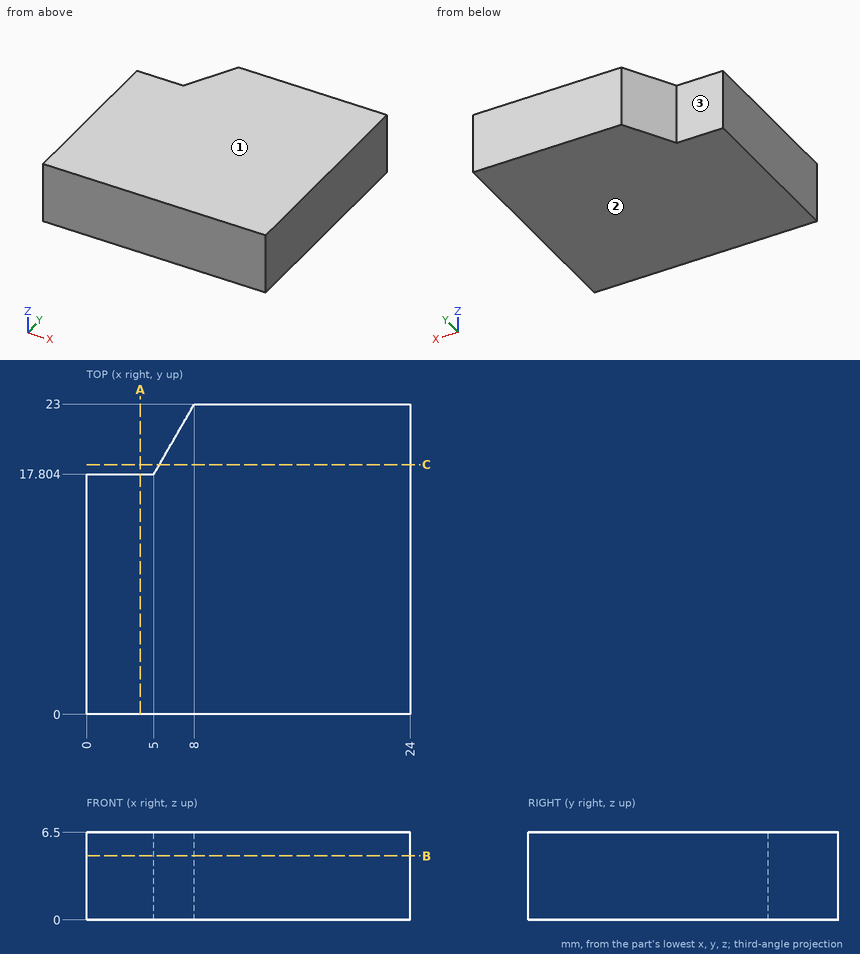
Verification items for this drawing (mm, ordinates from the low corner). Give positions to 0.01 mm unless a question says otherwise; leave off trailing zeros. Loops run counter-clockwise (first coordinate to the right, second up) from the corner with the lowest first, then second, coordinate; pieces in that order, holes last.
(1) Release check for a two-part mould opening along Z. For the marked faces 1, 2 and 3 record: released by +Z, released by -Z, zero draft, split by the parting line, or undercut.
From the geometry:
face 1: released by +Z
face 2: released by -Z
face 3: zero draft
(2) Section check C-C on y = 18.5. Record the cut outline in (x, z), then the cut area to 3 significant figures.
From the geometry:
outline: (5.4, 0) - (24, 0) - (24, 6.5) - (5.4, 6.5) - close
area: 121 mm2
(3) Section check A-A on x = 4. Record the cut outline in (y, z).
From the geometry:
outline: (0, 0) - (17.8, 0) - (17.8, 6.5) - (0, 6.5) - close
(4) Section check B-B on z = 4.75. Record the cut outline in (x, y).
From the geometry:
outline: (0, 0) - (24, 0) - (24, 23) - (8, 23) - (5, 17.8) - (0, 17.8) - close
(5) Depth check by flat-ended pin: pin 1 Ø12 at (x, y) = (19, 15) entering from -Z; pin 2 Ø2 at (y, z) = (20, 3) entering from -X. Enter the tip coordinate at first touch or a pass-through.
From the geometry:
pin 1: stops at z = 0
pin 2: stops at x = 5.69
(6) Thickness scan on L1, parallel to Y at x = 4.75, z = 2.25; L2, parallel to X at y = 19.5, z = 2.5; L3, parallel to Y at x = 7.75, z = 4. Record the ranges inside material, lowest first.
From the geometry:
L1: y = 0 to 17.8
L2: x = 5.98 to 24
L3: y = 0 to 22.57
